Input: part model. Units: mm. Frame: model coordinates. Face numbers are marked on the shaded views. A direction names the side the tool comes from. Coordinates: 2 decimals unless noted, no trailing zeros. Loops run counter-clockwise (first coordinate to the right, second up) from the corner with the lowest first, then second, coordinate; pieces in that order, holes last. Notation, with made-up numbers: (38, 75.5) - (63, 75.5) arc R11 ccw to (63, 94.5) - close; hole circle Ø5 at (28.5, 85). An arc over 180 degrees is marked (long way). Answer as CSV lines item,"result". Start each with the question number.
```python
from build123d import *

# Parameters (mm, degrees)
F2_R = 4.2248737342


with BuildPart() as f1:
    # F0 (on Front) → F1 (revolve)
    with BuildSketch(Plane.XZ):
        with BuildLine():
            Line((-9.2264421542, 14), (-5.05, 14))
            add(Edge.make_bspline(
                [(-5.05, 14), (-5.2072363825, 14.0810028272), (-7.9343017899, 13.3850205174), (-7.9161451117, 27.8848960237), (-7.9913089744, 29.7148263859), (-7.9540337168, 30.2082094767)],
                knots=[0, 0, 0, 0, 0.1839441933, 0.7528458391, 1, 1, 1, 1], degree=3))
            Line((-7.9540337168, 30.2082094767), (-7.9540337168, 39.2082094767))
            Line((-7.9540337168, 39.2082094767), (-9.9539440577, 39.2271469541))
            Line((-9.9539440577, 39.2271469541), (-9.9539440577, 30.2271469541))
            add(Edge.make_bspline(
                [(-9.2264421542, 14), (-9.3868926202, 14.0217893951), (-10.5124276426, 14.24964973), (-10.0890154715, 27.7222878167), (-10.0266310522, 30), (-9.9539440577, 30.2271469541)],
                knots=[0, 0, 0, 0, 0.1370918561, 0.7422285722, 1, 1, 1, 1], degree=3))
        make_face()
        with BuildLine():
            Line((-8.05, 0), (-5.05, 0))
            Line((-5.05, 0), (-5.05, 4))
            Line((-5.05, 4), (-4.75, 4))
            Line((-4.75, 4), (-4.75, 14))
            Line((-4.75, 14), (-5.05, 14))
            Line((-5.05, 14), (-9.2264421542, 14))
            Line((-9.2264421542, 14), (-9.2264421542, 2.4549234658))
            add(Edge.make_bspline(
                [(-19.05, 5.2343760617), (-18.8808851703, 4.2130953372), (-18.5850778449, 1.9601937624), (-12.7121775245, 1.892012544), (-10.6474171038, 2.2360002455), (-9.2264421542, 2.4549234658)],
                knots=[0, 0, 0, 0, 0.2839843179, 0.664766452, 1, 1, 1, 1], degree=3))
            Line((-19.05, 5.2343760617), (-19.05, 88))
            Line((-19.05, 88), (-21.05, 88))
            Line((-21.05, 88), (-21.05, 0))
            Line((-21.05, 0), (-8.05, 0))
        make_face()
    revolve(axis=Axis((0, 0, 10.4999532923), (0, 0, 1)))

    # F2
    f2_edges = [f1.edges().sort_by_distance(p)[0] for p in [
        (21.05, 0, 0),
    ]]
    fillet(f2_edges, radius=F2_R)


solid = f1.part
```
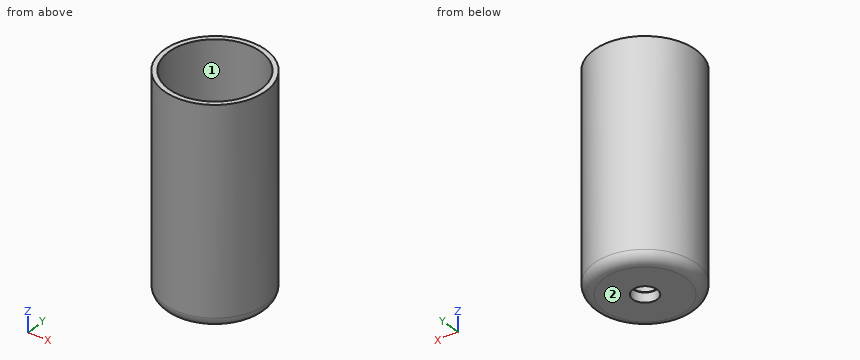
Item 1: Section query B-B, the plane z = 63. Output: boundary loops of the cut face in (x, y).
Item 2: Material intervals for probe 1 along X at (y, z) = (0, 33); probe 2 along X at (y, z) = (0, 10.25), sorted ascending.
Item 3: Section query A-A, the plane z = 38. Output: boundary loops of the cut face in (x, y), and give its area (3 significant figures).
Item 4: Set-up query: the marked faces 1 and 2. Return all of +Z, -Z, +X, -X, +Y, -Y with unobstructed straight access to the full face (end or side cutting, diameter ignored); none if empty.
Item 5: Section query C-C, the plane z = 24. Give the number of separate pieces and of enclosed holes in the cut face, and give its area (3 significant figures).
Item 6: Contact query for flat-ended pins moving along their axis: P1, Ø2, axis at x = -16.5, z = 74, coming from the -Y side; P2, Ø5, axis at x = 2, y = -9.5, coming from the +Z side; P3, Ø1.5, axis at y = 14.5, z = 35, coming from the +X side. Output: stop coordinate, or through.
Response values:
1,outline,"circle Ø42.1 at (0, 0); hole circle Ø38.1 at (0, 0)"
2,probe 1,"x = -21.05 to -19.05, -9.95 to -7.95, 7.95 to 9.95, 19.05 to 21.05"
2,probe 2,"x = -21.05 to -19.05, -9.23 to -4.75, 4.75 to 9.23, 19.05 to 21.05"
3,outline,"circle Ø42.1 at (0, 0); circle Ø19.91 at (0, 0); hole circle Ø38.1 at (0, 0); hole circle Ø15.91 at (0, 0)"
3,area,"364 mm²"
4,face 1,"+Z"
4,face 2,"-Z, +X, -X, +Y, -Y"
5,separate pieces,"2"
5,enclosed holes,"2"
5,area,"382 mm²"
6,P1,"stops at y = -14.24"
6,P2,"stops at z = 39.23"
6,P3,"stops at x = 15.94"
